Geometry check sheet. Reference: the model listing, model coordinates, mm. Round coordinates to 2 decimals unless told otherwise and drop trailing zeros. Order: outer loops, then holes, each group sorted by start corner. A loop starts at its lowest first (then second) coordinate and runs counter-clockwise, first axis right, second up.
(1) Thickness scan on L1, parallel to Z at x = 97.5, y = -0.35; L2, parallel to Z at x = -189, y = -1.2; L3, parallel to Z at x = 1.5, y = -1.2. Record the ranges inside material, lowest first.
(2) Gauge pin test, flat ends, axial feed: P1, Ø3, axis at x = 52.5, z = -2.5, coming from the -Y side; P2, Ø3.5, axis at x = 189, z = -40, coming from the -Y side. Record the tip position at first contact, or that the pin passes through.
(3) Cross-section at B-B on x = -25.5. Enter the section's corners in (y, z), and give its area (4 significant figures).
(4) Cross-section at A-A on x = 64. Enter the section's corners in (y, z).
(5) Cross-section at C-C on y = -1. Count the separate pieces of the cut face and the enclosed holes in it, and give its area (3 significant figures).
from build123d import *

# Parameters (mm, degrees)
F0_W     = 390
F0_H     = 120
F0_R     = 1.6
F0_R_2   = 4
F0_R_3   = 1.5
F0_R_4   = 7.5
F0_W_2   = 17.5
F0_H_2   = 5
F0_R_5   = 1.75
F0_W_3   = 50
F0_H_3   = 20
F0_R_6   = 2.5
F0_W_4   = 30
F0_H_4   = 2.5
F0_W_5   = 22.5
F0_W_6   = 45
F0_W_7   = 160
F0_R_7   = 4.75
F1_DEPTH = 1.8


with BuildPart() as f1:
    # F0 (on Front) → F1 (new body)
    with BuildSketch(Plane.XZ):
        Rectangle(F0_W, F0_H)
        with Locations((-113, -50)):
            Circle(F0_R, mode=Mode.SUBTRACT)
        with Locations((-189, -40)):
            Circle(F0_R, mode=Mode.SUBTRACT)
        with Locations((-172.5, -40)):
            Circle(F0_R_2, mode=Mode.SUBTRACT)
        with Locations((-135, -40)):
            Circle(F0_R_2, mode=Mode.SUBTRACT)
        with Locations((-108.6, -40)):
            Circle(F0_R_3, mode=Mode.SUBTRACT)
        with Locations((-36, -50)):
            Circle(F0_R, mode=Mode.SUBTRACT)
        with Locations((-97.5, -40)):
            Circle(F0_R_4, mode=Mode.SUBTRACT)
        with Locations((-86.4, -40)):
            Circle(F0_R_3, mode=Mode.SUBTRACT)
        with Locations((-78.6, -40)):
            Circle(F0_R_3, mode=Mode.SUBTRACT)
        with Locations((-67.5, -40)):
            Circle(F0_R_4, mode=Mode.SUBTRACT)
        with Locations((-56.4, -40)):
            Circle(F0_R_3, mode=Mode.SUBTRACT)
        with Locations((-172.5, -22.5)):
            Rectangle(F0_W_2, F0_H_2, mode=Mode.SUBTRACT)
        with Locations((-135, -22.5)):
            Rectangle(F0_W_2, F0_H_2, mode=Mode.SUBTRACT)
        with Locations((-172.5, -7.5)):
            Circle(F0_R_5, mode=Mode.SUBTRACT)
        with Locations((-135, -7.5)):
            Circle(F0_R_2, mode=Mode.SUBTRACT)
        with Locations((-97.5, -17.5)):
            Circle(F0_R_5, mode=Mode.SUBTRACT)
        with Locations((-67.5, -17.5)):
            Circle(F0_R_5, mode=Mode.SUBTRACT)
        with Locations((-41, -26.25)):
            Circle(F0_R_3, mode=Mode.SUBTRACT)
        with Locations((-97.5, -2.5)):
            Circle(F0_R_5, mode=Mode.SUBTRACT)
        with Locations((-67.5, -2.5)):
            Circle(F0_R_5, mode=Mode.SUBTRACT)
        with Locations((-20, -10)):
            Rectangle(F0_W_3, F0_H_3, mode=Mode.SUBTRACT)
        with Locations((44, -50)):
            Circle(F0_R, mode=Mode.SUBTRACT)
        with Locations((52.5, -32.5)):
            Circle(F0_R_5, mode=Mode.SUBTRACT)
        with Locations((75, -32.5)):
            Circle(F0_R_5, mode=Mode.SUBTRACT)
        with Locations((123, -50)):
            Circle(F0_R, mode=Mode.SUBTRACT)
        with Locations((97.5, -32.5)):
            Circle(F0_R_5, mode=Mode.SUBTRACT)
        with Locations((120, -32.5)):
            Circle(F0_R_5, mode=Mode.SUBTRACT)
        with Locations((142.5, -32.5)):
            Circle(F0_R_5, mode=Mode.SUBTRACT)
        with Locations((189, -40)):
            Circle(F0_R, mode=Mode.SUBTRACT)
        with Locations((175, -32.5)):
            Circle(F0_R_5, mode=Mode.SUBTRACT)
        with Locations((4, -26.25)):
            Circle(F0_R_3, mode=Mode.SUBTRACT)
        with Locations((52.5, -17.5)):
            Circle(F0_R_5, mode=Mode.SUBTRACT)
        with Locations((75, -17.5)):
            Circle(F0_R_5, mode=Mode.SUBTRACT)
        with Locations((22.5, -2.5)):
            Circle(F0_R_5, mode=Mode.SUBTRACT)
        with Locations((52.5, -2.5)):
            Circle(F0_R_5, mode=Mode.SUBTRACT)
        with Locations((75, -2.5)):
            Circle(F0_R_5, mode=Mode.SUBTRACT)
        with Locations((97.5, -17.5)):
            Circle(F0_R_5, mode=Mode.SUBTRACT)
        with Locations((120, -17.5)):
            Circle(F0_R_5, mode=Mode.SUBTRACT)
        with Locations((142.5, -17.5)):
            Circle(F0_R_5, mode=Mode.SUBTRACT)
        with Locations((175, -17.5)):
            Circle(F0_R_5, mode=Mode.SUBTRACT)
        with Locations((97.5, -2.5)):
            Circle(F0_R_5, mode=Mode.SUBTRACT)
        with Locations((120, -2.5)):
            Circle(F0_R_5, mode=Mode.SUBTRACT)
        with Locations((142.5, -2.5)):
            Circle(F0_R_5, mode=Mode.SUBTRACT)
        with Locations((175, -2.5)):
            Circle(F0_R_5, mode=Mode.SUBTRACT)
        with Locations((-172.5, 2.5)):
            Circle(F0_R_5, mode=Mode.SUBTRACT)
        with Locations((-172.5, 12.5)):
            Circle(F0_R_5, mode=Mode.SUBTRACT)
        with Locations((-135, 10)):
            Rectangle(F0_W_2, F0_H_2, mode=Mode.SUBTRACT)
        with Locations((-172.5, 22.5)):
            Circle(F0_R_5, mode=Mode.SUBTRACT)
        with Locations((-85, 15)):
            Circle(F0_R_6, mode=Mode.SUBTRACT)
        with Locations((-79.9, 15)):
            Circle(F0_R_6, mode=Mode.SUBTRACT)
        with Locations((-82.5, 28.75)):
            Rectangle(F0_W_4, F0_H_4, mode=Mode.SUBTRACT)
        with Locations((-20, 20)):
            Rectangle(F0_W_3, F0_H_3, mode=Mode.SUBTRACT)
        with Locations((-172.5, 32.5)):
            Circle(F0_R_5, mode=Mode.SUBTRACT)
        with Locations((-189, 40)):
            Circle(F0_R, mode=Mode.SUBTRACT)
        with Locations((-135, 30)):
            Circle(F0_R_2, mode=Mode.SUBTRACT)
        with Locations((-135, 47.5)):
            Rectangle(F0_W_5, F0_H_2, mode=Mode.SUBTRACT)
        with Locations((-113, 56)):
            Circle(F0_R, mode=Mode.SUBTRACT)
        with Locations((-82.5, 38.75)):
            Rectangle(F0_W_6, F0_H_4, mode=Mode.SUBTRACT)
        with Locations((-41, 36.25)):
            Circle(F0_R_3, mode=Mode.SUBTRACT)
        with Locations((-82.5, 48.75)):
            Rectangle(F0_W_6, F0_H_4, mode=Mode.SUBTRACT)
        with Locations((22.5, 12.5)):
            Circle(F0_R_5, mode=Mode.SUBTRACT)
        with Locations((52.5, 12.5)):
            Circle(F0_R_5, mode=Mode.SUBTRACT)
        with Locations((75, 12.5)):
            Circle(F0_R_5, mode=Mode.SUBTRACT)
        with Locations((97.5, 12.5)):
            Circle(F0_R_5, mode=Mode.SUBTRACT)
        with Locations((120, 12.5)):
            Circle(F0_R_5, mode=Mode.SUBTRACT)
        with Locations((142.5, 12.5)):
            Circle(F0_R_5, mode=Mode.SUBTRACT)
        with Locations((175, 12.5)):
            Circle(F0_R_5, mode=Mode.SUBTRACT)
        with Locations((175, 27.5)):
            Circle(F0_R_3, mode=Mode.SUBTRACT)
        with Locations((4, 36.25)):
            Circle(F0_R_3, mode=Mode.SUBTRACT)
        with Locations((50, 48.75)):
            Rectangle(F0_W_7, F0_H_4, mode=Mode.SUBTRACT)
        with Locations((175, 40)):
            Circle(F0_R_7, mode=Mode.SUBTRACT)
        with Locations((189, 40)):
            Circle(F0_R, mode=Mode.SUBTRACT)
        with Locations((123, 56)):
            Circle(F0_R, mode=Mode.SUBTRACT)
        with Locations((175, 52.5)):
            Circle(F0_R_3, mode=Mode.SUBTRACT)
    extrude(amount=F1_DEPTH)


solid = f1.part
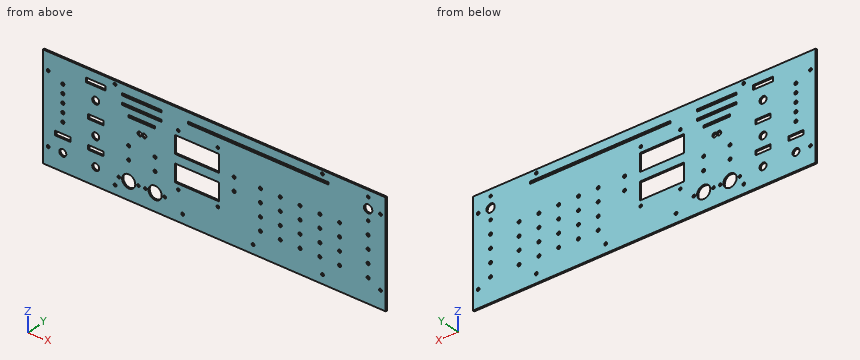
Found:
1. L1: z = -60 to -34.25, -30.75 to -19.25, -15.75 to -4.25, -0.75 to 10.75, 14.25 to 47.5, 50 to 60
1. L2: z = -60 to -41.6, -38.4 to 38.4, 41.6 to 60
1. L3: z = -60 to -20, 0 to 10, 30 to 47.5, 50 to 60
2. P1: passes through
2. P2: stops at y = -1.8
3. outline: (-1.8, -60) - (0, -60) - (0, -20) - (-1.8, -20) - close; (-1.8, 0) - (0, 0) - (0, 10) - (-1.8, 10) - close; (-1.8, 30) - (0, 30) - (0, 47.5) - (-1.8, 47.5) - close; (-1.8, 50) - (0, 50) - (0, 60) - (-1.8, 60) - close
3. area: 139.5 mm2
4. outline: (-1.8, -60) - (0, -60) - (0, 47.5) - (-1.8, 47.5) - close; (-1.8, 50) - (0, 50) - (0, 60) - (-1.8, 60) - close
5. separate pieces: 1
5. enclosed holes: 74
5. area: 42,600 mm2
